Autodesk Inventor part; units mm, degrees
ref_plane "YZ Plane" through (0, 0, 0) normal (1, 0, 0) x (0, 1, 0)
ref_plane "XZ Plane" through (0, 0, 0) normal (0, 1, 0) x (-1, 0, 0)
ref_plane "XY Plane" through (0, 0, 0) normal (0, 0, 1) x (1, 0, 0)
sketch "Sketch2" plane through (0, 0, 0) normal (0, 0, 1) x (1, 0, 0)
  line L0 (-105, -72.5) -> (105, -72.5)
  line L1 (105, -72.5) -> (105, 72.5)
  line L2 (105, 72.5) -> (-105, 72.5)
  line L3 (-105, 72.5) -> (-105, -72.5)
  line L4 (-105, -72.5) -> (105, 72.5) construction
  line L5 (105, -72.5) -> (-105, 72.5) construction
  point P0 (0, 0)
  dimension "d11" = 145
  dimension "d12" = 210
extrude "Extrusion2" add sketch "Sketch2" along normal blind 8
sketch "Sketch3" plane through (0, 0, 8) normal (0, 0, 1) x (1, 0, 0)
  line L0 (105, 72.5) -> (-105, 72.5)
  line L1 (-63, 72.5) -> (-21, 72.5)
  line L2 (-21, 72.5) -> (-21, 80.5)
  line L3 (-21, 80.5) -> (-63, 80.5)
  line L4 (-63, 80.5) -> (-63, 72.5)
  line L5 (63, 72.5) -> (21, 72.5)
  line L6 (21, 72.5) -> (21, 80.5)
  line L7 (21, 80.5) -> (63, 80.5)
  line L8 (63, 80.5) -> (63, 72.5)
  line L9 (-21, 80.5) -> (21, 80.5) construction
  line L10 (63, 80.5) -> (105, 80.5) construction
  line L11 (-63, 80.5) -> (-105, 80.5) construction
  point P0 (0, 0)
  dimension "d15" = 8
extrude "Extrusion3" add sketch "Sketch3" against normal blind 8
mirror "Mirror1" about plane through (0, 0, 0) normal (0, 1, 0) of "Extrusion3"
sketch "Sketch4" plane through (0, 0, 8) normal (0, 0, 1) x (1, 0, 0)
  line L0 (-105, 72.5) -> (-105, -72.5)
  line L1 (-105, -72.5) -> (-97, -72.5)
  line L2 (-97, -72.5) -> (-97, -24.1667)
  line L3 (-97, -24.1667) -> (-105, -24.1667)
  line L4 (-105, -24.1667) -> (-105, -72.5)
  line L5 (-105, 72.5) -> (-97, 72.5)
  line L6 (-97, 72.5) -> (-97, 24.1667)
  line L7 (-97, 24.1667) -> (-105, 24.1667)
  line L8 (-105, 24.1667) -> (-105, 72.5)
  line L9 (-97, -24.1667) -> (-97, 24.1667) construction
  point P0 (0, 0)
  dimension "d21" = 8
extrude "Extrusion4" cut sketch "Sketch4" against normal blind 8
mirror "Mirror2" about plane through (0, 0, 0) normal (1, 0, 0) of "Extrusion4"
properties part number "M06 - Wall Side 1" material "Wood (Walnut)"
Can you work these out from the model? Positions are in its coordinate system, mm. A direction names the side the tool comes from. Round coordinates to 2 decimals unless told otherwise and drop trailing zeros. Loops run counter-clockwise (first coordinate to the right, second up) from the corner with the lowest first, then second, coordinate; pieces in that order, holes last. Notation, with made-up numbers: M 21,50 L 38,50 A25 cw 38,82 Z; hole C 35.5,52.25 d1. An arc over 180 degrees is marked long. Answer in a Markdown table with one row per item.
1. I'm going to push flat-ended pins straight in: pin 1 Ø2.5 at (x, z) = (81.5, 2.5) entering from +Y; pin 2 Ø2.5 at (y, z) = (37.5, 5.5) entering from -X; pin 3 Ø4 at (x, z) = (-103, 6) entering from -Y. Where does each tip first touch, or does it pass through?
Established:
| item | result |
|---|---|
| pin 1 | y = 72.5 |
| pin 2 | x = -97 |
| pin 3 | y = -24.17 |
2. On a 3-axis mill with a long thin cutter (end or side, diameter ignored), from which of +Z, -Z, +X, -X, +Y, -Y can I reach the whole of each face in a straight line? I mean faces 4 (the face through (21, -77, 4)), 5 (the face through (97, 48, 4)), 6 (the face through (63, -76, 4)), 7 (the face through (-80, -72.5, 4)). Say none if no direction works.
Established:
| item | result |
|---|---|
| face 4 | +Z, -Z, -Y |
| face 5 | +Z, -Z, +X, +Y |
| face 6 | +Z, -Z, +X, -Y |
| face 7 | +Z, -Z, -X, -Y |
3. If we section it at A-A, the plane z = 4.25: Please give me the cut outline in (x, y), plus the area to 3 significant figures.
Established:
| item | result |
|---|---|
| outline | M -105,-24.17 L -97,-24.17 L -97,-72.5 L -63,-72.5 L -63,-80.5 L -21,-80.5 L -21,-72.5 L 21,-72.5 L 21,-80.5 L 63,-80.5 L 63,-72.5 L 97,-72.5 L 97,-24.17 L 105,-24.17 L 105,24.17 L 97,24.17 L 97,72.5 L 63,72.5 L 63,80.5 L 21,80.5 L 21,72.5 L -21,72.5 L -21,80.5 L -63,80.5 L -63,72.5 L -97,72.5 L -97,24.17 L -105,24.17 Z |
| area | 30,200 mm² |
4. If we section it at C-C, the plane y = 54: Please give me the cut outline in (x, z), plus the area to 3 significant figures.
Established:
| item | result |
|---|---|
| outline | M -97,0 L 97,0 L 97,8 L -97,8 Z |
| area | 1,550 mm² |
5. Thinking about a two-plate mould opening in X: for faces 1 (the face through (-42, -80.5, 4)), 2 (the face through (105, 0, 4)), 3 (the face through (-21, -77, 4)), which applies, pulls with the +X half, pulls with the -X half, needs draft (parallel to the pull), parting line crosses it, or undercut?
Established:
| item | result |
|---|---|
| face 1 | needs draft |
| face 2 | pulls with the +X half |
| face 3 | undercut |
6. Please list where these lines run through material, in increasing order: line 1 (X direction, y = -52, z = 5.25); line 2 (Y direction, x = 68.5, z = 4). Write a range as from..to.
Established:
| item | result |
|---|---|
| line 1 | -97..97 |
| line 2 | -72.5..72.5 |
7. If we section it at B-B, the plane x = -74.5: Please give me the cut outline in (y, z), plus the area to 3 significant figures.
Established:
| item | result |
|---|---|
| outline | M -72.5,0 L 72.5,0 L 72.5,8 L -72.5,8 Z |
| area | 1,160 mm² |
